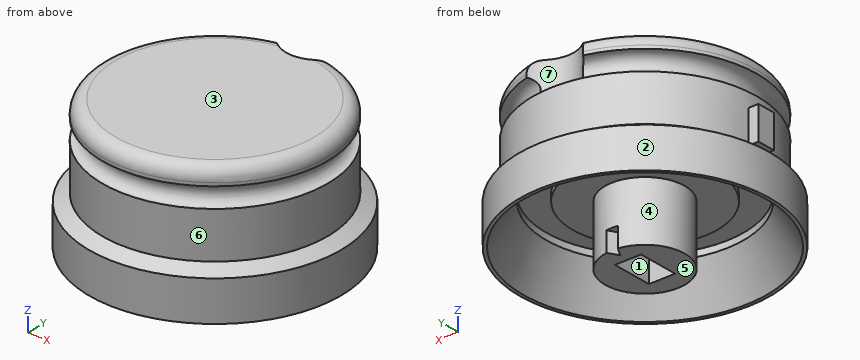
```python
from build123d import *

# Parameters (mm, degrees)
SKETCH064_W     = 6.2
SKETCH064_H     = 4
POCKET005_DEPTH = 4.2
SKETCH093_W     = 3
SKETCH093_H     = 2.8
PAD011_DEPTH    = 5
SKETCH101_R     = 5
POCKET022_DEPTH = 5.5
POCKET055_DEPTH = 3


with BuildPart() as part:
    # Sketch063 → Revolution016 (revolve)
    with BuildSketch(Plane.YZ):
        with BuildLine():
            Line((6.05, 9), (11, 9))
            Line((11, 9), (11, 10))
            Line((11, 10), (15, 10))
            Line((15, 10), (15, 9))
            Line((15, 9), (18.5, 2.937822))
            Line((18.5, 2.937822), (19, 2.937822))
            Line((19, 9), (19, 2.937822))
            Line((17, 10.154701), (19, 9))
            Line((17, 17.154701), (17, 10.154701))
            ThreePointArc((17, 20.154701), (15.5, 18.654701), (17, 17.154701))
            Line((17, 20.654701), (17, 20.154701))
            ThreePointArc((17, 20.654701), (16.414214, 22.068914), (15, 22.654701))
            Line((0, 22.654701), (15, 22.654701))
            Line((0, 22.654701), (0, 0))
            Line((0, 0), (6.05, 0))
            Line((6.05, 0), (6.05, 9))
        make_face()
    revolve(axis=Axis((0, 0, 0), (0, 0, 1)))

    # Sketch064 (on Face1 of Revolution016) → Pocket005 (cut)
    with BuildSketch(Plane.YX):
        Rectangle(SKETCH064_W, SKETCH064_H)
    extrude(amount=-POCKET005_DEPTH, mode=Mode.SUBTRACT)

    # Sketch093 → Pad011 (join)
    with BuildSketch(Plane.XY.offset(10)):
        with Locations((-17, 0)):
            Rectangle(SKETCH093_W, SKETCH093_H)
    extrude(amount=PAD011_DEPTH)

    # Sketch101 (on Face25 of Pad011) → Pocket022 (cut)
    with BuildSketch(Plane(origin=(0, 0, 22.654701), x_dir=(0, -1, 0), z_dir=(0, 0, 1))):
        with Locations((-19, 0)):
            Circle(SKETCH101_R)
    extrude(amount=-POCKET022_DEPTH, mode=Mode.SUBTRACT)

    # Sketch174 (on Face1 of Revolution016) → Pocket055 (cut)
    with BuildSketch(Plane.YX):
        Polygon((6.75, 1.299038), (4.5, 0), (6.75, -1.299038), align=None)
    extrude(amount=-POCKET055_DEPTH, mode=Mode.SUBTRACT)


with BuildPart() as part_1:
    # Body017 placement: moved
    add(part.part.moved(Location((0, 0, 80))))


solid = part_1.part
```
The model under review builds one solid part; all positions refer to its coordinate system, in mm. Face numbers are marked on the shaded views. A direction names the side the tool comes from. Round coordinates to 2 decimals unless told otherwise and drop trailing zeros. Order: outer loops, then holes, each group sorted by start corner. A loop starts at its lowest first (then second) coordinate and runs counter-clockwise, first axis right, second up.
Item 1: Machinability: for the marked faces 4, 5, 6 and 7, which of the approach directions +Z, -Z, +X, -X, +Y, -Y give a long, thin tool a straight path to every point of the face, cutting with its end or side? Answer none if there is none.
Working result:
face 4: -Z
face 5: -Z, +X, -X, +Y, -Y
face 6: +Z
face 7: +Z, +Y
Item 2: Add section C-C, the plane z = 97.75. State the section outline as (x, y) points.
Working result:
outline: (-3.48, 15.41) arc R15.8 ccw (long way) to (3.48, 15.41) arc R5 cw to start
Item 3: Draft analysis for pull direction Y (two halves, no side actions). For the marked faces 1, 2 and 3, state which applies: released by +Y, released by -Y, zero draft, split by the parting line, or undercut.
Working result:
face 1: undercut
face 2: split by the parting line
face 3: zero draft
Item 4: Add section B-B, the plane y = 15.5. Count the separate pieces of the cut face and the enclosed holes in it, and give its area (3 significant figures).
Working result:
separate pieces: 3
enclosed holes: 0
area: 198 mm2
Item 5: For pin 1 (2 mm diameter, centred on x = 0, y = -0.5, fed in from -Z); pin 2 (8 mm diameter, centred on x = 13.5, z = 83, fed in from +Y); pin 3 (1 mm diameter, centred on x = -14, y = -7, fed in from -Z), all flat-tipped, find the tip position at first contact; note any pin that passes through.
Working result:
pin 1: stops at z = 84.2
pin 2: stops at y = 16.45
pin 3: stops at z = 87
Item 6: To check wall thickness, follow probe 1 along X at (y, z) = (0, 89.25); probe 2 along Y at (x, z) = (0, 89.7); probe 3 along Y at (x, z) = (2, 88.25). State the ranges of each line that lie inside material, in increasing order.
Working result:
probe 1: x = -18.57 to -15, -11 to 11, 15 to 18.57
probe 2: y = -17.79 to -15, -11 to 11, 15 to 17.79
probe 3: y = -18.89 to -15.3, -5.71 to 5.71, 15.3 to 18.89
Item 7: Add section A-A, the plane z = 85. State the section outline as (x, y) points, and give its area (3 significant figures).
Working result:
outline: circle Ø38 at (0, 0); circle Ø12.1 at (0, 0); hole circle Ø34.62 at (0, 0)
area: 308 mm2
